Autodesk Inventor part; units mm, degrees
ref_plane "YZ Plane" through (0, 0, 0) normal (1, 0, 0) x (0, 1, 0)
ref_plane "XZ Plane" through (0, 0, 0) normal (0, 1, 0) x (-1, 0, 0)
ref_plane "XY Plane" through (0, 0, 0) normal (0, 0, 1) x (1, 0, 0)
sketch "Sketch1" plane through (0, 0, 0) normal (0, 1, 0) x (-1, 0, 0)
  line L0 (0, 0) -> (22.8388, 0)
  line L1 (22.8388, 0) -> (22.8388, -52)
  line L2 (22.8388, -52) -> (0, -52)
  line L3 (0, -52) -> (0, 0)
  line L4 (9, 0) -> (9, -16.4645)
  line L5 (12, -24.5962) -> (12, -35.182)
  line L6 (9, -28) -> (0, -28)
  line L7 (12, -35.182) -> (13.4142, -35.182)
  line L8 (13.4142, -35.182) -> (19.7782, -28.818)
  line L9 (19.7782, -28.818) -> (20.8388, -29.8787)
  line L10 (20.8388, -29.8787) -> (12, -38.7175)
  line L11 (12, -38.7175) -> (12, -52)
  line L12 (16.5962, -32) -> (17.6569, -33.0607) construction
  line L13 (16.5962, -32) -> (0, -32) construction
  line L14 (9, -16.4645) -> (9, -28)
  line L15 (20.8388, -29.8787) -> (19.7782, -28.818)
  line L16 (12, -24.5962) -> (21.1924, -15.4038)
  line L17 (16.5962, -32) -> (16.5962, -20) construction
  line L18 (16.5962, -20) -> (9, -20) construction
  line L19 (21.1924, -15.4038) -> (22.8388, -13.7574)
  line L20 (20.8388, -29.8787) -> (22.8388, -27.8787)
  line L21 (19.7782, -28.818) -> (22.8388, -25.7574)
  dimension "d8" = 9
  dimension "d9" = 1.5
  dimension "d10" = 8
  dimension "d11" = 20
  dimension "d12" = 12
  dimension "d18" = 28
  dimension "d46" = 45
  dimension "d48" = 3
  dimension "d49" = 45
  dimension "d50" = 2
  dimension "d51" = 4
  dimension "d52" = 20
extrude "Extrusion2" add sketch "Sketch1" along normal blind 20 contours L0 L1 L19 L16 L5 L7 L8 L9 L10 L11 L2 L3 L6 L14 L4 | L1 L20 L9 L21
sketch "Sketch3" plane through (-9, 0, 0) normal (1, 0, 0) x (0, 0, -1)
  line L0 (0, 0) -> (0, 20)
  line L1 (23.5, 13.5) -> (16.5, 13.5)
  line L2 (16.5, 13.5) -> (16.5, 6.5)
  line L3 (16.5, 6.5) -> (23.5, 6.5)
  line L4 (23.5, 6.5) -> (23.5, 13.5)
  circle A0 centre (5, 8) radius 1.397
  point P0 (16.5, 10)
  point P1 (16.5, 10)
  point P2 (0, 10)
  point P3 (20, 0)
  point P4 (20, 0)
  point P5 (20, 0)
  point P6 (20, 6.5)
  point P7 (0, 10)
  dimension "d19" = 2.794
  dimension "d20" = 5
  dimension "d33" = 2
  dimension "d53" = 7
extrude "Extrusion3" cut sketch "Sketch3" against normal up to next
sketch "Sketch4" plane through (0, 0, -28) normal (1, 0, 0) x (0, 0, -1)
  line L0 (24, 0) -> (24, 20)
  circle A0 centre (19, 8) radius 1.397
  circle A1 centre (4, 10) radius 2
  circle A2 centre (4, 10) radius 1.05
  point P0 (-28, 0)
  point P1 (24, 10)
  point P2 (24, 10)
  dimension "d23" = 2.794
  dimension "d24" = 4
  dimension "d25" = 2.1
  dimension "d26" = 5
  dimension "d27" = 2
  dimension "d28" = 20
extrude "Extrusion4" cut sketch "Sketch4" against normal up to next contours A0 | A2
extrude "Extrusion5" cut sketch "Sketch4" against normal blind 9 contours A1
sketch "Sketch5" plane through (-20.8388, 0, -29.8787) normal (-0.7071068, 0, -0.7071068) x (-0.7071068, 0, 0.7071068)
  ellipse E0 centre (-7.75, 10) end of major axis (-7.75, 11.05) minor radius 0.7425
  line L0 (-10.5, 4) -> (1.5, 4) construction
  line L1 (1.5, 4) -> (1.5, 16) construction
  line L2 (1.5, 16) -> (-10.5, 16) construction
  line L3 (-10.5, 16) -> (-10.5, 4) construction
  circle A0 centre (-10.5, 16) radius 0.5
  circle A1 centre (-10.5, 4) radius 0.5
  line L4 (-9, 5.5) -> (5.0245, 5.5)
  line L5 (5.0245, 5.5) -> (5.0245, 21.8088)
  line L6 (5.0245, 21.8088) -> (-9, 21.8088)
  line L7 (-9, 21.8088) -> (-9, 5.5)
  circle A2 centre (1.5, 4) radius 0.5
  point P0 (6.3921, 0)
  point P1 (-4.5, 0)
  point P2 (-4.5, 0)
  point P3 (-4.5, 0)
  point P4 (-10.5, 10)
  point P5 (-4.5, 4)
  point P6 (-4.5, 10)
  dimension "d35" = 12
  dimension "d37" = 1
  dimension "d40" = 4.5
  dimension "d41" = 4.5
extrude "Extrusion6" cut sketch "Sketch5" against normal blind 3.5 contours E0 | A0 | A1 | L7 L6 L5 L4 | A2
extrude "Extrusion1" add sketch "Sketch1" against normal blind 3
chamfer "Chamfer1" distance 2.54 angle 45 4 edges at (-22.8388, -3, -26) (-11.4194, -3, -52) (-11.4194, -3, 0) (0, -3, -26)
properties part number "minimal micro scanner"
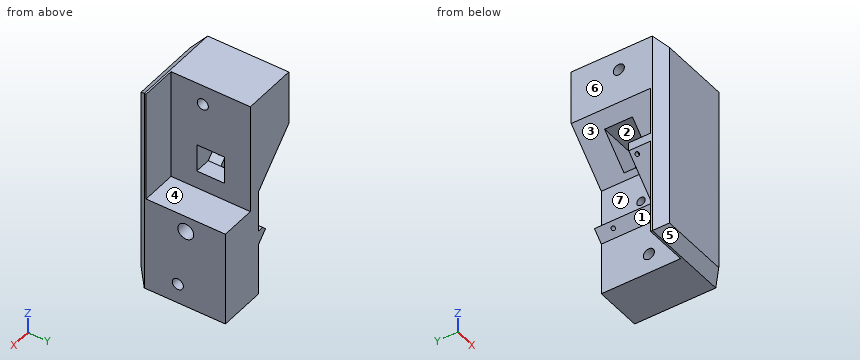
Check sheet for the modelled part. Datum: model origin and axes. Units: mm. Face numbers are marked on the shaded views. A direction names the side the tool comes from. Give positions to 0.01 mm unless a question says otherwise; leave off trailing zeros. Order: outer loops, then holes, each group sorted by start corner. A loop starts at its lowest first (then second) coordinate and runs counter-clockwise, first axis right, second up. Notation, with made-up numbers: (23, 56) -> (77, 56) arc R18 ccw to (77, 60) -> close; hole circle Ø11 at (5.25, 14.5). An arc over 180 degrees is marked (long way). Return JSON: item names as keys, results as strings.
1. Set-up check for the marked faces 1, 2, 3 and 4: record each of +Z, -Z, +X, -X, +Y, -Y from which the full face is reachable in a straight line by a thin tool's end or side.
From the geometry:
{"face 1": "-Z, -X, +Y", "face 2": "+X, -X", "face 3": "-X, +Y", "face 4": "+Z, +X, +Y"}
2. Mould release check, pull along X, two halves, no side actions. Record for the marked faces 5, 6 and 7: +X half, -X half, draft (parallel to the pull), parting line (faces both ways), or undercut.
From the geometry:
{"face 5": "draft", "face 6": "-X half", "face 7": "undercut"}
3. Cross-section at A-A, the plane y = 10. Count the separate pieces of the cut face and the enclosed holes in it, plus the area to 3 significant figures.
From the geometry:
{"separate pieces": "3", "enclosed holes": "0", "area": "490 mm^2"}
4. Cross-section at C-C, the plane x = -19.5. Record the cut outline in (y, z), plus the area to 3 significant figures.
From the geometry:
{"outline": "(-3, -49.46) -> (-0.46, -52) -> (0, -52) -> (0, -31.22) -> (5.5, -31.22) -> (5.5, -29.1) -> (0, -29.1) -> (0, -17.1) -> (6.5, -17.1) -> (6.5, -16.5) -> (13.5, -16.5) -> (13.5, -17.1) -> (20, -17.1) -> (20, 0) -> (-0.46, 0) -> (-3, -2.54) -> close; hole circle Ø2.79 at (8, -5)", "area": "493 mm^2"}
5. Material ranges on probe 1 along Y at (x, z) = (-7, -32); probe 2 along Y at (x, z) = (-11.3, -32); probe 3 along Y at (x, z) = (-8.5, -23), recorded low to high. Write a range as [from, to].
From the geometry:
{"probe 1": "[-3, 8], [12, 20]", "probe 2": "[-3, 8.95], [11.05, 20]", "probe 3": "[-3, 0]"}
6. Go/stop test with flat-tipped pins: P1, Ø5, axis at y = 5.5, z = -34.5, coming from the +X side; P2, Ø10.5, axis at x = -18.5, z = -28.5, coming from the +Y side; P3, Ø1.2, axis at y = 10.5, z = -32.5, coming from the +X side; P4, Ø2.5, axis at y = 8, z = -47, coming from the +X side. Record where each tip stops, or that it passes through.
From the geometry:
{"P1": "x = 0", "P2": "y = 5.5", "P3": "x = -9", "P4": "through"}
7. Cross-section at B-B, the plane z = -47. Record the cut outline in (x, y), plus the area to 3 significant figures.
From the geometry:
{"outline": "(-22.84, -0.46) -> (-20.3, -3) -> (-2.54, -3) -> (0, -0.46) -> (0, 6.6) -> (-12, 6.6) -> (-12, 0) -> (-22.84, 0) -> close; (-12, 9.4) -> (0, 9.4) -> (0, 20) -> (-12, 20) -> close", "area": "269 mm^2"}
